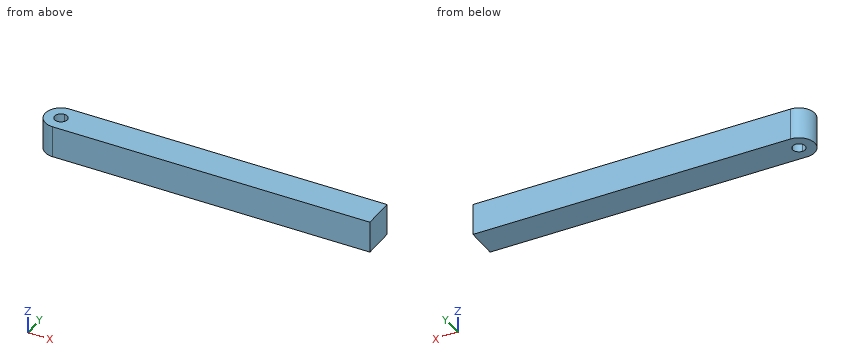
```python
from build123d import *

# Parameters (mm, degrees)
EXTRUDE_1_DEPTH = 100


with BuildPart() as part:
    # ｽｹｯﾁ1 → ﾎﾞｽ - 押し出し1 (new body)
    with BuildSketch(Plane.XY):
        with BuildLine():
            ThreePointArc((-500, 50), (-550, 0), (-500, -50))
            Line((-500, -50), (-500, -20))
            ThreePointArc((-500, -20), (-520, 0), (-500, 20))
            Line((-500, 20), (-500, 50))
        make_face()
        with BuildLine():
            Line((-500, -20), (-500, -50))
            ThreePointArc((-500, -50), (-464.644660941, -35.355339059), (-450, 0))
            ThreePointArc((-450, 0), (-464.644660941, 35.355339059), (-500, 50))
            Line((-500, 50), (-500, 20))
            ThreePointArc((-500, 20), (-485.857864376, 14.142135624), (-480, 0))
            ThreePointArc((-480, 0), (-485.857864376, -14.142135624), (-500, -20))
        make_face()
        with BuildLine():
            ThreePointArc((-450, 0), (-464.644660941, -35.355339059), (-500, -50))
            Line((-500, -50), (500, -50))
            Line((500, -50), (500, 50))
            Line((500, 50), (-500, 50))
            ThreePointArc((-500, 50), (-464.644660941, 35.355339059), (-450, 0))
        make_face()
    extrude(amount=EXTRUDE_1_DEPTH)


solid = part.part
```
Read the model definition and answer for the solid it produces. Units are mm, in the model's axes. Give positions to 0.01 mm unless a question says otherwise; leave off trailing zeros. Order: outer loops, then holes, each group sorted by start corner. A loop starts at its lowest first (then second) coordinate and runs counter-clockwise, first axis right, second up.
(1) Straight lines are drawn through the part: L1, parallel to X at y = 25.5, z = 64.5; L2, parallel to X at y = -16, z = 49; L3, parallel to X at y = 28, z = 22.5. For each, find the intervals that lie inside material, in ascending order.
(2) Given pin 1 (6 mm diameter, centred on y = 24, z = 51.5, fed in from -X); pin 2 (10 mm diameter, centred on y = 1, z = 44, fed in from -X); pin 3 (1 mm diameter, centred on y = 25.5, z = 37, fed in from -X), each flat-ended and moving along its own axis, determine where each tip first touches the part or whether it passes through.
(3) Find section A-A (z = 14). Give the vertices of the cut face in (x, y).
(4) Find section B-B (y = -37). Give the vertices of the cut face in (x, z).
Result sheet:
1. L1: x = -543.01 to 500
1. L2: x = -547.37 to -512, -488 to 500
1. L3: x = -541.42 to 500
2. pin 1: stops at x = -545.38
2. pin 2: stops at x = -550
2. pin 3: stops at x = -543.3
3. outline: (-500, -50) - (500, -50) - (500, 50) - (-500, 50) arc R50 ccw to start; hole circle Ø40 at (-500, 0)
4. outline: (-533.63, 0) - (500, 0) - (500, 100) - (-533.63, 100) - close
